Work out the finished part from the listing and answer in its coordinate system (mm). A direction names the side the tool comes from. Give positions to 0.01 mm unless a question says otherwise; leave off trailing zeros. Loops run counter-clockwise (first coordinate to the right, second up) from the corner with the lowest first, then second, coordinate; pieces in that order, holes last. Notation, with made-up numbers: (1, 46) - (54, 46) arc R20 ccw to (54, 69) - close; hole circle Ø11 at (56.5, -25.5). An arc over 180 degrees is marked (long way). One line per item, written item: value.
from build123d import *

# Parameters (mm, degrees)
SKETCH1_R           = 1.5
SKETCH1_W           = 42
SKETCH1_H           = 21
BOSS_EXTRUDE1_DEPTH = 5
FILLET2_R           = 10
FILLET3_R           = 10


with BuildPart() as part:
    # Sketch1 → Boss-Extrude1 (new body)
    with BuildSketch(Plane.XY):
        Polygon((-28.086956522, 0), (-17.269090954, 0), (-17.269090954, -5), (-4.269090954, -5), (-4.269090954, 0), (-0.586956522, 0), (-0.586956522, -5), (12.413043478, -5), (12.413043478, 0), (16.095177911, 0), (16.095177911, -5), (29.095177911, -5), (29.095177911, 0), (39.913043478, 0), (39.913043478, 33), (-28.086956522, 33), align=None)
        with Locations((30.413043478, 21.75)):
            Circle(SKETCH1_R, mode=Mode.SUBTRACT)
        with Locations((30.413043478, 11.75)):
            Circle(SKETCH1_R, mode=Mode.SUBTRACT)
        with Locations((-17.586956522, 21.75)):
            Circle(SKETCH1_R, mode=Mode.SUBTRACT)
        with Locations((-17.586956522, 11.75)):
            Circle(SKETCH1_R, mode=Mode.SUBTRACT)
        with Locations((5.913043478, 16.5)):
            Rectangle(SKETCH1_W, SKETCH1_H, mode=Mode.SUBTRACT)
    extrude(amount=BOSS_EXTRUDE1_DEPTH)

    # Fillet2
    fillet2_edges = [part.edges().sort_by_distance(p)[0] for p in [
        (-28.086956522, 33, 2.5),
    ]]
    fillet(fillet2_edges, radius=FILLET2_R)

    # Fillet3
    fillet3_edges = [part.edges().sort_by_distance(p)[0] for p in [
        (39.913043478, 33, 2.5),
    ]]
    fillet(fillet3_edges, radius=FILLET3_R)


solid = part.part
1. For faces 5 (the flat face through (6, 27, 2)), 6 (the flat face through (-0.587, -2, 2)), 7 (the flat face through (34, 0, 2)), 8 (the flat face through (-11, -5, 2)), determine the directions among +Z, -Z, +X, -X, +Y, -Y from which every point of the face is accessible in a straight line to the end or side of a thin tool.
Output:
face 5: +Z, -Z
face 6: +Z, -Z, -Y
face 7: +Z, -Z, +X, -Y
face 8: +Z, -Z, +X, -X, -Y
2. Flat-ended cylindrical pins translate along their axes: pin 1 Ø5 at (x, y) = (-17.59, 21.75) entering from -Z; pin 2 Ø1.5 at (y, z) = (-2.5, 1.5) entering from -X; pin 3 Ø1.5 at (y, z) = (-3, 2.5) entering from +X. Find the tip coordinate at first contact, or state that the pin passes through.
Output:
pin 1: stops at z = 0
pin 2: stops at x = -17.27
pin 3: stops at x = 29.1
3. Section B-B (z = 3) is taken. Write down the section's boundary in (x, y), and give its area (3 significant figures).
Output:
outline: (-28.09, 0) - (-17.27, 0) - (-17.27, -5) - (-4.27, -5) - (-4.27, 0) - (-0.59, 0) - (-0.59, -5) - (12.41, -5) - (12.41, 0) - (16.1, 0) - (16.1, -5) - (29.1, -5) - (29.1, 0) - (39.91, 0) - (39.91, 23) arc R10 ccw to (29.91, 33) - (-18.09, 33) arc R10 ccw to (-28.09, 23) - close; hole circle Ø3 at (-17.59, 11.75); hole circle Ø3 at (-17.59, 21.75); hole (-15.09, 6) - (26.91, 6) - (26.91, 27) - (-15.09, 27) - close; hole circle Ø3 at (30.41, 11.75); hole circle Ø3 at (30.41, 21.75)
area: 1,490 mm²
4. The mould has two halves that part along X. Classify faces 1 (the cylindrical face through (-25.24, 29.99, 2.54)), 2 (the cylindrical face through (36.906, 30.148, 2.535)), 3 (the flat face through (12.413, -3, 2)), 4 (the flat face through (14, 0, 2)): released by +X, released by -X, zero draft, split by the parting line, or undercut.
Output:
face 1: released by -X
face 2: released by +X
face 3: undercut
face 4: undercut
5. Section C-C (x = -13.5) is taken. Write down the section's boundary in (y, z).
Output:
outline: (-5, 0) - (6, 0) - (6, 5) - (-5, 5) - close; (27, 0) - (33, 0) - (33, 5) - (27, 5) - close
6. Find the intervals of material crossed by line 1 along X through (y, z) = (-1, 3.35); line 2 along X through (y, z) = (10, 0.65); line 3 along Y through (x, z) = (-5.5, 4.4), in increasing order.
Output:
line 1: x = -17.27 to -4.27, -0.59 to 12.41, 16.1 to 29.1
line 2: x = -28.09 to -15.09, 26.91 to 39.91
line 3: y = -5 to 6, 27 to 33
7. Section A-A (y = 18.5) is taken. Write down the section's boundary in (x, z).
Output:
outline: (-28.09, 0) - (-15.09, 0) - (-15.09, 5) - (-28.09, 5) - close; (26.91, 0) - (39.91, 0) - (39.91, 5) - (26.91, 5) - close
8. Section D-D (y = 11.75) is taken. Write down the section's boundary in (x, z).
Output:
outline: (-28.09, 0) - (-19.09, 0) - (-19.09, 5) - (-28.09, 5) - close; (-16.09, 0) - (-15.09, 0) - (-15.09, 5) - (-16.09, 5) - close; (26.91, 0) - (28.91, 0) - (28.91, 5) - (26.91, 5) - close; (31.91, 0) - (39.91, 0) - (39.91, 5) - (31.91, 5) - close
